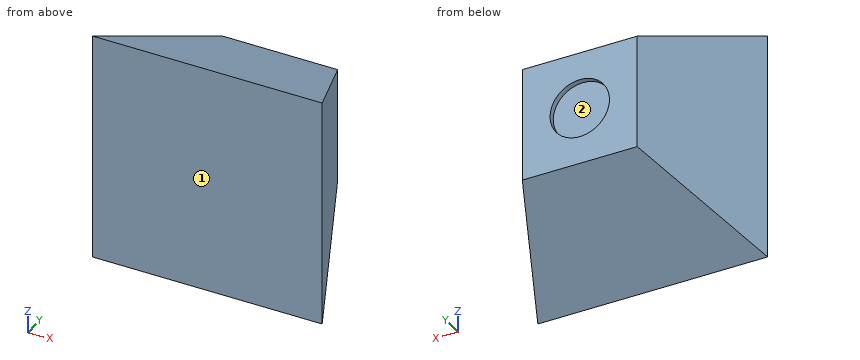
```python
from build123d import *

# Parameters (mm, degrees)
SKETCH_3_R          = 15.5
CUT_EXTRUDE_1_DEPTH = 3


with BuildPart() as part:
    # 草图2 → 放样1 section 0
    with BuildSketch(Plane(origin=(0, 70, 0), x_dir=(1, 0, 0), z_dir=(0, 1, 0))):
        with BuildLine():
            Line((-30, -30), (30, -30))
            Line((30, -30), (30, 30))
            Line((30, 30), (-30, 30))
            Line((-30, 30), (-30, -30))
        make_face()
    # 草图1 → 放样1 section 1
    with BuildSketch(Plane(origin=(0, 0, 0), x_dir=(1, 0, 0), z_dir=(0, 1, 0))):
        with BuildLine():
            Line((-60, -60), (60, -60))
            Line((60, -60), (60, 60))
            Line((60, 60), (-60, 60))
            Line((-60, 60), (-60, -60))
        make_face()
    loft()

    # 草图3 → 切除-拉伸1 (cut)
    with BuildSketch(Plane(origin=(0, 70, 0), x_dir=(1, 0, 0), z_dir=(0, 1, 0))):
        with Locations(Location((0, 0, 0), (0, 0, 270))):
            Circle(SKETCH_3_R)
    extrude(amount=-CUT_EXTRUDE_1_DEPTH, mode=Mode.SUBTRACT)


solid = part.part
```
Source: CAD feature listing. Evaluate the final solid. Frame: model axes, mm. Face numbers are marked on the shaded views. Give positions to 0.01 mm unless a question says otherwise; leave off trailing zeros. Use a Markdown table: item, result.
Q1. First-contact query: P1, Ø8, axis at y = 16.5, z = 40, coming from the +X side; P2, Ø1.5, axis at x = 23.5, z = 34.5, coming from the -Y side; P3, Ø6, axis at y = 10, z = -17, coming from the +X side; P4, Ø1.5, axis at y = 31, z = -40, coming from the +X side. Flat tips, straight axial feed; report the tip coordinate or a pass-through.
A:
| item | result |
|---|---|
| P1 | x = 54.64 |
| P2 | y = 0 |
| P3 | x = 57 |
| P4 | x = 47.04 |
Q2. Material intervals for line 1 (Y direction, x = 0.5, z = 12); line 2 (X direction, y = 68, z = 0); line 3 (X direction, y = 69.25, z = 0), sorted ascending. Write a range as [from, to].
A:
| item | result |
|---|---|
| line 1 | [0, 67] |
| line 2 | [-30.86, -15.5], [15.5, 30.86] |
| line 3 | [-30.32, -15.5], [15.5, 30.32] |
Q3. Pull-direction query (X, two-part tool) for the marked faces 1 and 2; classes: +X half, -X half, draft (parallel to the pull), parting line (faces both ways), or undercut.
A:
| item | result |
|---|---|
| face 1 | draft |
| face 2 | undercut |
